Geometry: final body of the model. Coordinates: model frame, mm. A direction names the side the tool comes from. Coordinates: 2 decimals unless noted, no trailing zeros. Order: outer loops, then holes, each group sorted by start corner. A loop starts at its lowest first (then second) coordinate and runs counter-clockwise, first axis right, second up. Notation, with made-up numbers: M 36.5,51.5 L 85.5,51.5 A19 ccw 85.5,74.5 Z; hole C 25,-21.5 d7. An arc over 180 degrees is marked long. Use CSV: the item, a comma, the result in double quotes. Start each with the question number.
Q1. Section query D-D, the plane y = 15. Output: boundary loops of the cut face in (x, z) (3 decimals), and give its area (3 significant figures).
Q2. Mould query, pull axis Y, two halves, no side actions, for faces 6 (the face through (0, 30, 46)), 7 (the face through (-25, 15, -12)), 8 (the face through (0, 0, 180)). Classes: +Y half, -Y half, draft (parallel to the pull), parting line (faces both ways), or undercut.
Q3. First-contact query: P1, Ø16.5, axis at x = -1.5, z = 35, coming from the +Y side; P2, Ø4, axis at x = -12, z = 122.5, coming from the -Y side; P3, Ø4, axis at x = 9.5, z = 88, coming from the -Y side; P4, Ø4, axis at x = 18.5, y = 10.5, coming from the -Z side. Flat tips, straight axial feed; report the tip coordinate or a pass-through.
Q4. Section query C-C, the plane x = 21. Output: boundary loops of the cut face in (y, z), and give its area (3 significant figures).
Q5. Ray query, probe 1 along Z at (x, y) = (0.5, 23.5); probe 2 along Y at (x, z) = (2, 72); probe 3 along Z at (x, y) = (2, 36). Return the intervals inside material, ascending.
Q6. Access query for faces 1 (the face through (0, -5, 159.755)), 2 (the face through (-16.585, 15, -4)), 3 (the face through (20.9, 20.1, -7)), 4 (the face through (5.5, 15, 168)), 5 (the face through (0, 15, 169.755)). Directions: +Z, -Z, +X, -X, +Y, -Y. A direction counts if a zero-diameter tool reaches every point of the face in a straight line with its end or side. Return the directions, or none.
Q7. Section query B-B, the plane z = -12.5. Output: boundary loops of the cut face in (x, y) (3 decimals).
Q8. Section query A-A, the plane y = 26.5. Output: boundary loops of the cut face in (x, z) (3 decimals).
from build123d import *

# Parameters (mm, degrees)
BOSS_EXTRUDE2_DEPTH = 30
SKETCH4_R           = 7.5
BOSS_EXTRUDE3_DEPTH = 25
BOSS_EXTRUDE4_DEPTH = 5.5


with BuildPart() as part:
    # Sketch1 → Boss-Extrude2 (new body)
    with BuildSketch(Plane(origin=(0, 0, 0), x_dir=(1, 0, 0), z_dir=(0, 1, 0))):
        Polygon((-16.585, 0), (-5.986840434, -159.755193945), (5.986840434, -159.755193945), (16.585, 0), (16.585, 25), (-16.585, 25), align=None)
    extrude(amount=BOSS_EXTRUDE2_DEPTH)

    # Sketch4 → Boss-Extrude3 (add, symmetric)
    with BuildSketch(Plane(origin=(0, 0, 0), x_dir=(0, 0, -1), z_dir=(1, 0, 0))):
        with Locations((12.5, 15)):
            Circle(SKETCH4_R)
    extrude(amount=BOSS_EXTRUDE3_DEPTH, both=True)

    # Sketch6 → Boss-Extrude4 (add, symmetric)
    with BuildSketch(Plane(origin=(0, 0, 0), x_dir=(0, 0, -1), z_dir=(1, 0, 0))):
        Polygon((-189.755193945, 40), (-159.755193945, 40), (-159.755193945, -10), (-189.755193945, -10), (-189.755193945, 0), (-169.755193945, 0), (-169.755193945, 30), (-189.755193945, 30), align=None)
    extrude(amount=BOSS_EXTRUDE4_DEPTH, both=True)


solid = part.part
Responses:
1,outline,"M -25,-20 L -16.585,-20 L -16.585,-25 L 16.585,-25 L 16.585,-20 L 25,-20 L 25,-5 L 16.585,-5 L 16.585,0 L 5.987,159.755 L 5.5,159.755 L 5.5,169.755 L -5.5,169.755 L -5.5,159.755 L -5.987,159.755 L -16.585,0 L -16.585,-5 L -25,-5 Z"
1,area,"4,800 mm²"
2,face 6,"+Y half"
2,face 7,"draft"
2,face 8,"undercut"
3,P1,"stops at y = 30"
3,P2,"passes through"
3,P3,"stops at y = 0"
3,P4,"stops at z = -25"
4,outline,"C 15,-12.5 d15"
4,area,"177 mm²"
5,probe 1,"z = -25 to 169.76"
5,probe 2,"y = 0 to 30"
5,probe 3,"z = 159.76 to 189.76"
6,face 1,"-Z, +X, -X, -Y"
6,face 2,"-X"
6,face 3,"+X"
6,face 4,"+Z, +X, +Y, -Y"
6,face 5,"+Z, +X, -X"
7,outline,"M -25,7.5 L -16.585,7.5 L -16.585,0 L 16.585,0 L 16.585,7.5 L 25,7.5 L 25,22.5 L 16.585,22.5 L 16.585,30 L -16.585,30 L -16.585,22.5 L -25,22.5 Z"
8,outline,"M -16.585,-25 L 16.585,-25 L 16.585,0 L 5.987,159.755 L 5.5,159.755 L 5.5,169.755 L -5.5,169.755 L -5.5,159.755 L -5.987,159.755 L -16.585,0 Z"
